Can you work these out from the model? Positions are in its coordinate system, mm. Face numbers are marked on the shaded views. A direction names the side the tool comes from. Round coordinates to 2 decimals unless told otherwise and drop trailing zeros. Order: outer loops, then holes, each group sorted by start corner. A loop starts at its lowest first (then second) coordinate and runs counter-clockwise, first axis right, second up.
from build123d import *

# Parameters (mm, degrees)
BOSS_EXTRUDE1_DEPTH = 30
SKETCH1_3_R         = 56
SKETCH1_3_R_2       = 38
BOSS_EXTRUDE2_DEPTH = 50
SKETCH1_4_R         = 75
BOSS_EXTRUDE3_DEPTH = 40
SKETCH1_5_R         = 37.5
SKETCH1_5_R_2       = 18
BOSS_EXTRUDE4_DEPTH = 70


with BuildPart() as part:
    # Sketch1 → Boss-Extrude1 (new body)
    with BuildSketch(Plane(origin=(0, 0, 0), x_dir=(1, 0, 0), z_dir=(0, 1, 0))):
        with BuildLine():
            Line((-215, 66.580778007), (-215, 112.5))
            ThreePointArc((-215, 112.5), (-271, 56.5), (-327, 112.5))
            Line((-327, 112.5), (-327, -112.5))
            ThreePointArc((-327, -112.5), (-271, -56.5), (-215, -112.5))
            Line((-215, -112.5), (-215, -66.580778007))
            ThreePointArc((-215, -66.580778007), (-199.097061097, -47.83489279), (-178.009661836, -60.469498866))
            ThreePointArc((-178.009661836, -60.469498866), (0, -188), (178.009661836, -60.469498866))
            ThreePointArc((178.009661836, -60.469498866), (199.097061097, -47.83489279), (215, -66.580778007))
            Line((215, -66.580778007), (215, -112.5))
            ThreePointArc((215, -112.5), (271, -56.5), (327, -112.5))
            Line((327, -112.5), (327, 112.5))
            ThreePointArc((327, 112.5), (271, 56.5), (215, 112.5))
            Line((215, 112.5), (215, 66.580778007))
            ThreePointArc((215, 66.580778007), (199.097061097, 47.83489279), (178.009661836, 60.469498866))
            ThreePointArc((178.009661836, 60.469498866), (0, 188), (-178.009661836, 60.469498866))
            ThreePointArc((-178.009661836, 60.469498866), (-199.097061097, 47.83489279), (-215, 66.580778007))
        make_face()
        with BuildLine():
            ThreePointArc((121.794279026, 36.222216668), (154.328550802, 29.750752398), (169, 0))
            ThreePointArc((169, 0), (154.328553545, -29.750750294), (121.794285703, -36.222218458))
            ThreePointArc((121.794285703, -36.222218458), (87.408455986, -50.465295497), (92.266504099, -87.365836108))
            ThreePointArc((92.266504099, -87.365836108), (100.395482416, -99.531711756), (103.25, -113.882340598))
            ThreePointArc((103.25, -113.882340598), (70.644732229, -151.061522896), (29.527781525, -123.58805483))
            ThreePointArc((29.527781525, -123.58805483), (1.17e-07, -100.930591138), (-29.527781464, -123.588054603))
            ThreePointArc((-29.527781464, -123.588054603), (-84.499999831, -146.358293337), (-92.266504435, -87.365836444))
            ThreePointArc((-92.266504435, -87.365836444), (-87.408455896, -50.465295654), (-121.794285812, -36.222218487))
            ThreePointArc((-121.794285812, -36.222218487), (-169, -7.12e-07), (-121.794287187, 36.222218855))
            ThreePointArc((-121.794287187, 36.222218855), (-87.408455347, 50.465296604), (-92.266506993, 87.365839002))
            ThreePointArc((-92.266506993, 87.365839002), (-84.499998373, 146.358294179), (-29.527781529, 123.588054845))
            ThreePointArc((-29.527781529, 123.588054845), (1.47e-07, 100.930591138), (29.527781605, 123.58805513))
            ThreePointArc((29.527781605, 123.58805513), (70.644732383, 151.061522876), (103.25, 113.882340598))
            ThreePointArc((103.25, 113.882340598), (100.395482507, 99.531711976), (92.266504435, 87.365836444))
            ThreePointArc((92.266504435, 87.365836444), (87.408454139, 50.465298696), (121.794279026, 36.222216668))
        make_face(mode=Mode.SUBTRACT)
    extrude(amount=BOSS_EXTRUDE1_DEPTH)

    # Sketch1_3 → Boss-Extrude2 (add)
    # profile 1 of 4: a face of its own
    with BuildSketch(Plane(origin=(0, 0, 0), x_dir=(1, 0, 0), z_dir=(0, 1, 0))):
        with Locations((-271, 112.5)):
            Circle(SKETCH1_3_R)
        with Locations(Location((-271, 112.5, 0), (0, 0, 270))):
            Circle(SKETCH1_3_R_2, mode=Mode.SUBTRACT)
    # profile 2 of 4: a face of its own
    with BuildSketch(Plane(origin=(0, 0, 0), x_dir=(1, 0, 0), z_dir=(0, 1, 0))):
        with Locations(Location((-271, -112.5, 0), (0, 0, 180))):
            Circle(SKETCH1_3_R)
        with Locations(Location((-271, -112.5, 0), (0, 0, 270))):
            Circle(SKETCH1_3_R_2, mode=Mode.SUBTRACT)
    # profile 3 of 4: a face of its own
    with BuildSketch(Plane(origin=(0, 0, 0), x_dir=(1, 0, 0), z_dir=(0, 1, 0))):
        with Locations(Location((271, -112.5, 0), (0, 0, 180))):
            Circle(SKETCH1_3_R)
        with Locations(Location((271, -112.5, 0), (0, 0, 270))):
            Circle(SKETCH1_3_R_2, mode=Mode.SUBTRACT)
    # profile 4 of 4: a face of its own
    with BuildSketch(Plane(origin=(0, 0, 0), x_dir=(1, 0, 0), z_dir=(0, 1, 0))):
        with Locations((271, 112.5)):
            Circle(SKETCH1_3_R)
        with Locations(Location((271, 112.5, 0), (0, 0, 270))):
            Circle(SKETCH1_3_R_2, mode=Mode.SUBTRACT)
    extrude(amount=BOSS_EXTRUDE2_DEPTH)

    # Sketch1_4 → Boss-Extrude3 (add)
    with BuildSketch(Plane(origin=(0, 0, 0), x_dir=(1, 0, 0), z_dir=(0, 1, 0))):
        with BuildLine():
            ThreePointArc((121.794285703, -36.222218458), (94, -3.457e-06), (121.794279026, 36.222216668))
            ThreePointArc((121.794279026, 36.222216668), (87.408454139, 50.465298696), (92.266504435, 87.365836444))
            ThreePointArc((92.266504435, 87.365836444), (46.999999933, 81.406387994), (29.527781605, 123.58805513))
            ThreePointArc((29.527781605, 123.58805513), (1.47e-07, 100.930591138), (-29.527781529, 123.588054845))
            ThreePointArc((-29.527781529, 123.588054845), (-28.570817702, 118.777072835), (-28.25, 113.882340598))
            ThreePointArc((-28.25, 113.882340598), (-51.399373049, 79.236857398), (-92.266506993, 87.365839002))
            ThreePointArc((-92.266506993, 87.365839002), (-87.408455347, 50.465296604), (-121.794287187, 36.222218855))
            ThreePointArc((-121.794287187, 36.222218855), (-101.749250173, 22.828554154), (-94, 0))
            ThreePointArc((-94, 0), (-101.74924974, -22.828553589), (-121.794285812, -36.222218487))
            ThreePointArc((-121.794285812, -36.222218487), (-87.408455896, -50.465295654), (-92.266504435, -87.365836444))
            ThreePointArc((-92.266504435, -87.365836444), (-51.399371378, -79.23685809), (-28.25, -113.882340598))
            ThreePointArc((-28.25, -113.882340598), (-28.570817686, -118.777072711), (-29.527781464, -123.588054603))
            ThreePointArc((-29.527781464, -123.588054603), (1.17e-07, -100.930591138), (29.527781525, -123.58805483))
            ThreePointArc((29.527781525, -123.58805483), (46.999999862, -81.406388035), (92.266504099, -87.365836108))
            ThreePointArc((92.266504099, -87.365836108), (87.408455986, -50.465295497), (121.794285703, -36.222218458))
        make_face()
        with Locations(Location((0, 0, 0), (0, 0, 270))):
            Circle(SKETCH1_4_R, mode=Mode.SUBTRACT)
    extrude(amount=BOSS_EXTRUDE3_DEPTH)

    # Sketch1_5 → Boss-Extrude4 (add)
    # profile 1 of 6: a face of its own
    with BuildSketch(Plane(origin=(0, 0, 0), x_dir=(1, 0, 0), z_dir=(0, 1, 0))):
        with Locations(Location((65.75, 113.882340598, 0), (0, 0, 165))):
            Circle(SKETCH1_5_R)
        with Locations(Location((65.75, 113.882340598, 0), (0, 0, 270))):
            Circle(SKETCH1_5_R_2, mode=Mode.SUBTRACT)
    # profile 2 of 6: a face of its own
    with BuildSketch(Plane(origin=(0, 0, 0), x_dir=(1, 0, 0), z_dir=(0, 1, 0))):
        with Locations(Location((131.5, 0, 0), (0, 0, 105))):
            Circle(SKETCH1_5_R)
        with Locations(Location((131.5, 0, 0), (0, 0, 270))):
            Circle(SKETCH1_5_R_2, mode=Mode.SUBTRACT)
    # profile 3 of 6: a face of its own
    with BuildSketch(Plane(origin=(0, 0, 0), x_dir=(1, 0, 0), z_dir=(0, 1, 0))):
        with Locations(Location((65.75, -113.882340598, 0), (0, 0, 45))):
            Circle(SKETCH1_5_R)
        with Locations(Location((65.75, -113.882340598, 0), (0, 0, 270))):
            Circle(SKETCH1_5_R_2, mode=Mode.SUBTRACT)
    # profile 4 of 6: a face of its own
    with BuildSketch(Plane(origin=(0, 0, 0), x_dir=(1, 0, 0), z_dir=(0, 1, 0))):
        with Locations(Location((-65.75, -113.882340598, 0), (0, 0, 135))):
            Circle(SKETCH1_5_R)
        with Locations(Location((-65.75, -113.882340598, 0), (0, 0, 270))):
            Circle(SKETCH1_5_R_2, mode=Mode.SUBTRACT)
    # profile 5 of 6: a face of its own
    with BuildSketch(Plane(origin=(0, 0, 0), x_dir=(1, 0, 0), z_dir=(0, 1, 0))):
        with Locations(Location((-131.5, 0, 0), (0, 0, 75))):
            Circle(SKETCH1_5_R)
        with Locations(Location((-131.5, 0, 0), (0, 0, 270))):
            Circle(SKETCH1_5_R_2, mode=Mode.SUBTRACT)
    # profile 6 of 6: a face of its own
    with BuildSketch(Plane(origin=(0, 0, 0), x_dir=(1, 0, 0), z_dir=(0, 1, 0))):
        with Locations(Location((-65.75, 113.882340598, 0), (0, 0, 15))):
            Circle(SKETCH1_5_R)
        with Locations(Location((-65.75, 113.882340598, 0), (0, 0, 270))):
            Circle(SKETCH1_5_R_2, mode=Mode.SUBTRACT)
    extrude(amount=BOSS_EXTRUDE4_DEPTH)


solid = part.part
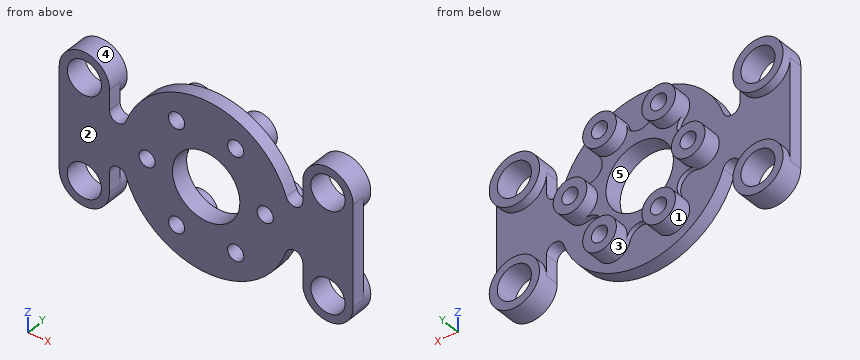
(1) I want a section at C-C, the plane x = 271. List the corners of the cut face in (y, z) for me.
(2) On a 3-axis mill with a long thin cutter (end or side, diameter ignored), from which of +Z, -Z, +X, -X, +Y, -Y can I reach the whole of each face in a straight line? I mean the marked faces 4 and 5. Say none if no direction works.
(3) I want a section at D-D, the plane x = 0. List the corners of the cut face in (y, z) for me, plus the area to 3 significant figures.
(4) If we mould it in two halves opening along Z, with no side actions, what happens to the marked faces 1, 2 and 3? For each: pulls with the +Z half, pulls with the -Z half, needs draft (parallel to the pull), parting line crosses it, or undercut.
(5) I want a section at A-A, the plane z = 0. List the corners of the cut face in (x, y) for me.
(6) Please list where these lines run through material, in increasing order: probe 1 along X at (y, z) = (18, 15.5); probe 2 along X at (y, z) = (4.5, -143); probe 3 along Z at (x, y) = (255.5, 47.5).
(7) I want a section at B-B, the plane y = 63. Give the number of separate pieces and of enclosed holes in the cut face, plus the area to 3 significant figures.
(8) I'm going to push flat-ended pins straight in: pin 1 Ø12 at (x, z) = (-86, -66.5) entering from +Y; pin 2 Ø1.5 at (x, y) = (-79, 45) entering from +Z; pin 3 Ø3 at (x, y) = (-84, 30.5) entering from -Z. Where does each tip first touch, or does it pass through?
Ans:
1. outline: (0, -168.5) - (50, -168.5) - (50, -150.5) - (0, -150.5) - close; (0, -74.5) - (50, -74.5) - (50, -56.5) - (30, -56.5) - (30, 56.5) - (50, 56.5) - (50, 74.5) - (0, 74.5) - close; (0, 150.5) - (50, 150.5) - (50, 168.5) - (0, 168.5) - close
2. face 4: +Y
2. face 5: +Y, -Y
3. outline: (0, -188) - (30, -188) - (30, -100.93) - (40, -100.93) - (40, -75) - (0, -75) - close; (0, 75) - (40, 75) - (40, 100.93) - (30, 100.93) - (30, 188) - (0, 188) - close
3. area: 7,300 mm2
4. face 1: undercut
4. face 2: needs draft
4. face 3: undercut
5. outline: (-327, 0) - (-149.5, 0) - (-149.5, 70) - (-169, 70) - (-169, 30) - (-327, 30) - close; (-113.5, 0) - (-75, 0) - (-75, 40) - (-94, 40) - (-94, 70) - (-113.5, 70) - close; (75, 0) - (113.5, 0) - (113.5, 70) - (94, 70) - (94, 40) - (75, 40) - close; (149.5, 0) - (327, 0) - (327, 30) - (169, 30) - (169, 70) - (149.5, 70) - close
6. probe 1: x = -327 to -140.65, -122.35 to -73.38, 73.38 to 122.35, 140.65 to 327
6. probe 2: x = -317.97 to -293.67, -248.33 to -224.03, -122.05 to 122.05, 224.03 to 248.33, 293.67 to 317.97
6. probe 3: z = -166.31 to -147.2, -77.8 to -58.69, 58.69 to 77.8, 147.2 to 166.31
7. separate pieces: 6
7. enclosed holes: 6
7. area: 20,400 mm2
8. pin 1: stops at y = 40
8. pin 2: stops at z = 149.24
8. pin 3: stops at z = -168.89
